For this review, use the dimensioned drawing (mm, ordinates from the lowest corner) and the shaded views. A direction names the side the tool comes from. Round coordinates to 2 decimals unless told otherwise and drop trailing zeros. Order: outer loops, then holes, each group sorted by start corner. A loop starts at its lowest first (then second) coordinate and runs counter-clockwise, first axis right, second up. Notation, with made-up numbers: M 75.25,-8 L 123.25,-8 A22 cw 123.25,6 Z; hole C 79.25,15 d1. An arc over 180 degrees is marked long. Use a Markdown table: item, result. Add a question column.
1. To check wall thickness, follow probe 1 along X at (y, z) = (14.5, 9.25) (1 decimal); probe 2 along Y at (x, z) = (31.5, 6.5); probe 3 along Y at (x, z) = (14, 15.5). State the ranges of each line that lie inside material, in increasing order.
2. Consider section C-C on x = 61.5. State the section outline as (y, z) points.
3. Insertion check: P1, Ø2, axis at x = 63, y = 32, coming from the +Z side; P2, Ø12, axis at x = 6, z = 11.5, coming from the +Y side; P3, Ø3, axis at y = 19, z = 13, coming from the -X side (3 decimals). Each pin has a flat end and moves straight along its axis. Give the tip position at first contact, or say it passes through.
4. Consider section A-A on z = 14. State the section outline as (x, y) points (1 decimal), then the cut area to 3 significant figures.
5. The part is to be moulded in two halves that separate along X. For the marked faces 1, 2 and 3, say which applies: +X half, -X half, draft (parallel to the pull), parting line (faces both ways), or undercut.
6. Consider section B-B on x = 75. State the section outline as (y, z) points.
7. For the marked faces 4, 5, 6 and 7, list the 3-axis set-ups (+Z, -Z, +X, -X, +Y, -Y) from which the entire face can be reached by the end or side of a thin tool; tool diameter is ignored.
8. Consider section D-D on y = 4. State the section outline as (x, z) points (3 decimals), then the cut area to 3 significant figures.
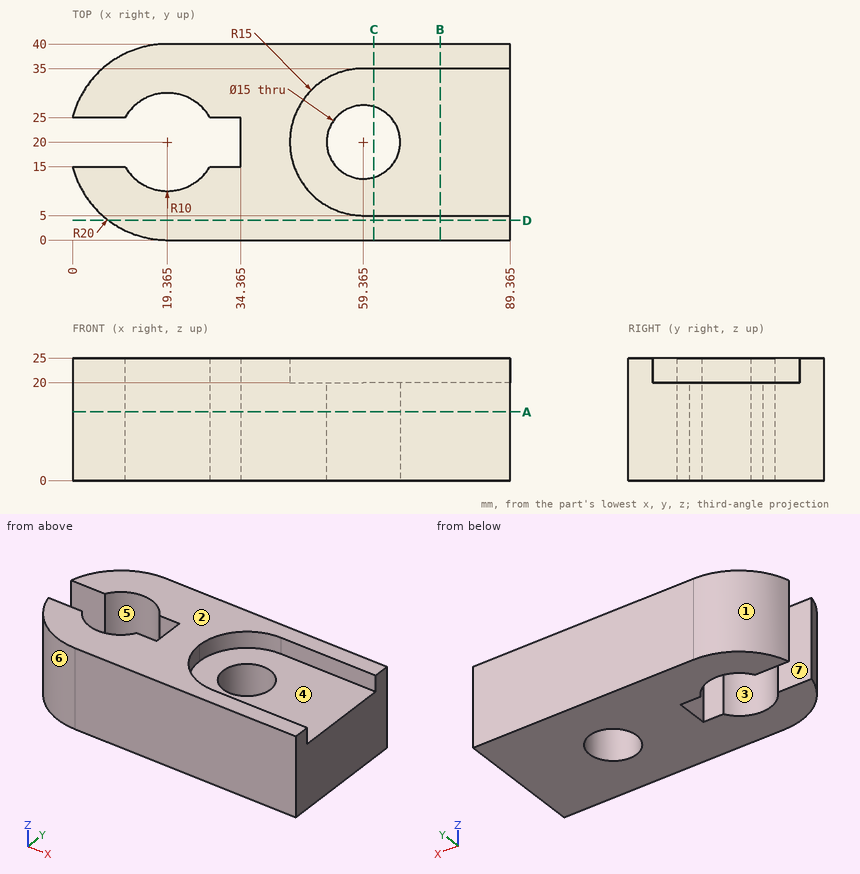
Answer block:
| question | item | result |
|---|---|---|
| 1 | probe 1 | 0.1 to 11, 27.7 to 54.3, 64.5 to 89.4 |
| 1 | probe 2 | 0 to 15, 25 to 40 |
| 1 | probe 3 | 0.73 to 11.56, 28.44 to 39.27 |
| 2 | outline | M 0,0 L 12.81,0 L 12.81,20 L 5,20 L 5,25 L 0,25 Z; M 27.19,0 L 40,0 L 40,25 L 35,25 L 35,20 L 27.19,20 Z |
| 3 | P1 | z = 20 |
| 3 | P2 | y = 38.59 |
| 3 | P3 | x = 34.365 |
| 4 | outline | M 0,15 A20 ccw 19.4,0 L 89.4,0 L 89.4,40 L 19.4,40 A20 ccw 0,25 L 10.7,25 A10 cw 28,25 L 34.4,25 L 34.4,15 L 28,15 A10 cw 10.7,15 Z; hole C 59.4,20 d15 |
| 4 | area | 2,780 mm^2 |
| 5 | face 1 | -X half |
| 5 | face 2 | draft |
| 5 | face 3 | undercut |
| 6 | outline | M 0,0 L 40,0 L 40,25 L 35,25 L 35,20 L 5,20 L 5,25 L 0,25 Z |
| 7 | face 4 | +Z, +X |
| 7 | face 5 | +Z, -Z |
| 7 | face 6 | +Z, -Z, -X, -Y |
| 7 | face 7 | +Z, -Z, -X |
| 8 | outline | M 7.365,0 L 89.365,0 L 89.365,25 L 7.365,25 Z |
| 8 | area | 2,050 mm^2 |
